Could you check a few things on this model? Use its own coordinates, in mm. A direction names the side the tool comes from. Round coordinates to 2 decimals unless told otherwise and drop trailing zeros. Loops run counter-clockwise (first coordinate to the right, second up) from the corner with the lowest first, then second, coordinate; pieces in that order, holes last. Notation, with made-up numbers: (37, -35) -> (82, -35) arc R10 ccw to (82, -22) -> close; hole circle Ø3 at (-34, 25.5). An arc over 180 degrees is marked (long way). One line per item, written item: value.
```python
from build123d import *

# Parameters (mm, degrees)
SKETCH1_W           = 500
SKETCH1_H           = 93
BOSS_EXTRUDE1_DEPTH = 3
SKETCH2_R           = 2.1
CUT_EXTRUDE1_DEPTH  = 255.305426604
LPATTERN1_COUNT     = 2
LPATTERN1_PITCH     = 70
FILLET1_R           = 10
CUT_EXTRUDE2_DEPTH  = 255.305426604
SKETCH4_R           = 2.1
CUT_EXTRUDE3_DEPTH  = 255.305426604


with BuildPart() as part:
    # Sketch1 → Boss-Extrude1 (new body)
    with BuildSketch(Plane.XY):
        Rectangle(SKETCH1_W, SKETCH1_H)
    extrude(amount=BOSS_EXTRUDE1_DEPTH)

    # Sketch2 → Cut-Extrude1 (cut, through all)
    with BuildSketch(Plane.XY.offset(3)):
        with Locations((-240, 33.5)):
            Circle(SKETCH2_R)
        with Locations((-160, 33.5)):
            Circle(SKETCH2_R)
        with Locations((-80, 33.5)):
            Circle(SKETCH2_R)
        with Locations((0, 33.5)):
            Circle(SKETCH2_R)
        with Locations((80, 33.5)):
            Circle(SKETCH2_R)
        with Locations((160, 33.5)):
            Circle(SKETCH2_R)
        with Locations((240, 33.5)):
            Circle(SKETCH2_R)
    cut_extrude1 = extrude(amount=-CUT_EXTRUDE1_DEPTH, mode=Mode.SUBTRACT)

    # LPattern1: Cut-Extrude1 ×2
    with Locations(*[(0, -i * LPATTERN1_PITCH, 0) for i in range(1, LPATTERN1_COUNT)]):
        add(cut_extrude1, mode=Mode.SUBTRACT)

    # Fillet1
    fillet1_edges = [part.edges().sort_by_distance(p)[0] for p in [
        (250, -46.5, 1.5),
        (-250, -46.5, 1.5),
        (-250, 46.5, 1.5),
        (250, 46.5, 1.5),
    ]]
    fillet(fillet1_edges, radius=FILLET1_R)

    # Sketch3 → Cut-Extrude2 (cut, through all)
    with BuildSketch(Plane.XY.offset(3)):
        with BuildLine():
            Line((-190, -17.393549254), (-190, 17.393549254))
            ThreePointArc((-190, 17.393549254), (-189.217522858, 18.980255935), (-187.48236191, 19.325400907))
            Line((-187.48236191, 19.325400907), (-122.568752369, 1.931851653))
            ThreePointArc((-122.568752369, 1.931851653), (-121.086390459, 0), (-122.568752369, -1.931851653))
            Line((-122.568752369, -1.931851653), (-187.48236191, -19.325400907))
            ThreePointArc((-187.48236191, -19.325400907), (-189.217522858, -18.980255935), (-190, -17.393549254))
        make_face()
        with BuildLine():
            Line((190, -17.393549254), (190, 17.393549254))
            ThreePointArc((190, 17.393549254), (189.217522858, 18.980255935), (187.48236191, 19.325400907))
            Line((187.48236191, 19.325400907), (122.568752369, 1.931851653))
            ThreePointArc((122.568752369, 1.931851653), (121.086390459, 0), (122.568752369, -1.931851653))
            Line((122.568752369, -1.931851653), (187.48236191, -19.325400907))
            ThreePointArc((187.48236191, -19.325400907), (189.217522858, -18.980255935), (190, -17.393549254))
        make_face()
    extrude(amount=-CUT_EXTRUDE2_DEPTH, mode=Mode.SUBTRACT)

    # Sketch4 → Cut-Extrude3 (cut, through all)
    with BuildSketch(Plane.XY.offset(3)):
        with Locations((-80, 0)):
            Circle(SKETCH4_R)
        with Locations((-60, 0)):
            Circle(SKETCH4_R)
        with Locations((-40, 0)):
            Circle(SKETCH4_R)
        with Locations((-20, 0)):
            Circle(SKETCH4_R)
        Circle(SKETCH4_R)
        with Locations(Location((20, 0, 0), (0, 0, 180))):
            Circle(SKETCH4_R)
        with Locations(Location((40, 0, 0), (0, 0, 180))):
            Circle(SKETCH4_R)
        with Locations(Location((60, 0, 0), (0, 0, 180))):
            Circle(SKETCH4_R)
        with Locations(Location((80, 0, 0), (0, 0, 180))):
            Circle(SKETCH4_R)
        with Locations((-80, -20)):
            Circle(SKETCH4_R)
        with Locations((-60, -20)):
            Circle(SKETCH4_R)
        with Locations((-40, -20)):
            Circle(SKETCH4_R)
        with Locations((-20, -20)):
            Circle(SKETCH4_R)
        with Locations((0, -20)):
            Circle(SKETCH4_R)
        with Locations(Location((20, -20, 0), (0, 0, 180))):
            Circle(SKETCH4_R)
        with Locations(Location((40, -20, 0), (0, 0, 180))):
            Circle(SKETCH4_R)
        with Locations(Location((60, -20, 0), (0, 0, 180))):
            Circle(SKETCH4_R)
        with Locations(Location((80, -20, 0), (0, 0, 180))):
            Circle(SKETCH4_R)
        with Locations((80, 20)):
            Circle(SKETCH4_R)
        with Locations((60, 20)):
            Circle(SKETCH4_R)
        with Locations((40, 20)):
            Circle(SKETCH4_R)
        with Locations((20, 20)):
            Circle(SKETCH4_R)
        with Locations(Location((0, 20, 0), (0, 0, 180))):
            Circle(SKETCH4_R)
        with Locations(Location((-20, 20, 0), (0, 0, 180))):
            Circle(SKETCH4_R)
        with Locations(Location((-40, 20, 0), (0, 0, 180))):
            Circle(SKETCH4_R)
        with Locations(Location((-60, 20, 0), (0, 0, 180))):
            Circle(SKETCH4_R)
        with Locations(Location((-80, 20, 0), (0, 0, 180))):
            Circle(SKETCH4_R)
    extrude(amount=-CUT_EXTRUDE3_DEPTH, mode=Mode.SUBTRACT)


solid = part.part
```
(1) Imagine slicing it at C-C on z = 0.8. Give the number of separate pieces and of enclosed holes in the cut face, then the cut area to 3 significant figures.
Results below:
separate pieces: 1
enclosed holes: 43
area: 42,900 mm²
(2) Imagine slicing it at A-A on y = -12. Write out the boundary of the cut face in (x, z), then the cut area to 3 significant figures.
Results below:
outline: (-250, 0) -> (-190, 0) -> (-190, 3) -> (-250, 3) -> close; (-160.14, 0) -> (160.14, 0) -> (160.14, 3) -> (-160.14, 3) -> close; (190, 0) -> (250, 0) -> (250, 3) -> (190, 3) -> close
area: 1,320 mm²
(3) On a 3-axis mill with a long thin cutter (end or side, diameter ignored), from which of +Z, -Z, +X, -X, +Y, -Y can I reach the whole of each face in a straight line? I mean faces 4 (the face through (246.99, 43.65, 1.52)), 5 (the face through (-155.48, 10.75, 1.52)). Say none if no direction works.
Results below:
face 4: +Z, -Z, +X, +Y
face 5: +Z, -Z
(4) Imagine slicing it at B-B on x = 179.5. Write out the boundary of the cut face in (y, z).
Results below:
outline: (-46.5, 0) -> (-17.19, 0) -> (-17.19, 3) -> (-46.5, 3) -> close; (17.19, 0) -> (46.5, 0) -> (46.5, 3) -> (17.19, 3) -> close
(5) Please list where these lines run through material, in increasing order: L1, parallel to Y at x = 40, z = 1.15; L2, parallel to Y at x = -240, z = 0.6; L3, parallel to Y at x = 41.5, z = 2.1.
Results below:
L1: y = -46.5 to -22.1, -17.9 to -2.1, 2.1 to 17.9, 22.1 to 46.5
L2: y = -46.5 to -38.6, -34.4 to 31.4, 35.6 to 46.5
L3: y = -46.5 to -21.47, -18.53 to -1.47, 1.47 to 18.53, 21.47 to 46.5
(6) For pin 1 Ø4 at (x, y) = (-80, 33.5) entering from +Z, with a flat end and sliding along its axis, tell me the tip position at first contact or that it passes through.
Results below:
pin 1: passes through
(7) We'd pull the mould along Y, two halves only. Please class faces 1 (the face through (-247.15, 43.49, 1.52)), 2 (the face through (-3, 1, 3)), 3 (the face through (155.48, 10.75, 1.52)): +Y half, -Y half, draft (parallel to the pull), parting line (faces both ways), or undercut.
Results below:
face 1: +Y half
face 2: draft
face 3: undercut
